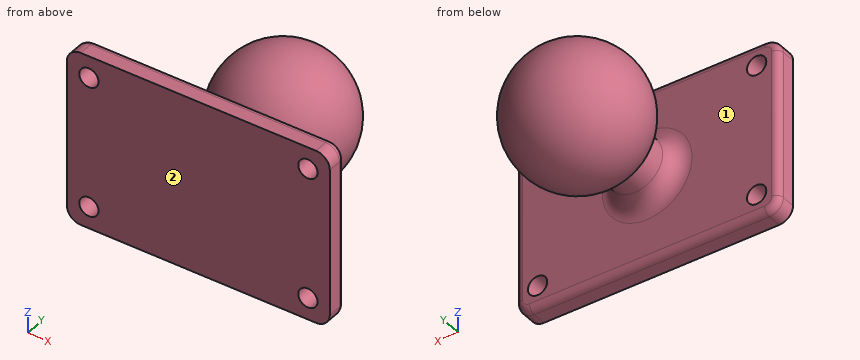
from build123d import *

# Parameters (mm, degrees)
SKETCH1_R           = 2.794
BOSS_EXTRUDE1_DEPTH = 6
FILLET1_R           = 5
FILLET2_R           = 2


with BuildPart() as part:
    # Sketch1 → Boss-Extrude1 (new body)
    with BuildSketch(Plane(origin=(0, 0, 0), x_dir=(1, 0, 0), z_dir=(0, 1, 0))):
        with BuildLine():
            Line((-34.1, -25.4), (34.1, -25.4))
            ThreePointArc((34.1, -25.4), (36.928427125, -24.228427125), (38.1, -21.4))
            Line((38.1, -21.4), (38.1, 21.4))
            ThreePointArc((38.1, 21.4), (36.928427125, 24.228427125), (34.1, 25.4))
            Line((34.1, 25.4), (-34.1, 25.4))
            ThreePointArc((-34.1, 25.4), (-36.928427125, 24.228427125), (-38.1, 21.4))
            Line((-38.1, 21.4), (-38.1, -21.4))
            ThreePointArc((-38.1, -21.4), (-36.928427125, -24.228427125), (-34.1, -25.4))
        make_face()
        with Locations(Location((-31.75, 19.05, 0), (0, 0, 270))):
            Circle(SKETCH1_R, mode=Mode.SUBTRACT)
        with Locations(Location((31.75, 19.05, 0), (0, 0, 270))):
            Circle(SKETCH1_R, mode=Mode.SUBTRACT)
        with Locations(Location((31.75, -19.05, 0), (0, 0, 270))):
            Circle(SKETCH1_R, mode=Mode.SUBTRACT)
        with Locations(Location((-31.75, -19.05, 0), (0, 0, 270))):
            Circle(SKETCH1_R, mode=Mode.SUBTRACT)
    extrude(amount=BOSS_EXTRUDE1_DEPTH)

    # Sketch2 → Revolve1 (revolve)
    with BuildSketch(Plane.XY, mode=Mode.PRIVATE) as revolve1_sk:
        with BuildLine():
            Line((0, 6), (0, 54.022796951))
            ThreePointArc((0, 54.022796951), (-18.604489806, 39.068582473), (-8, 17.684))
            Line((-8, 17.684), (-8, 6))
            Line((-8, 6), (0, 6))
        make_face()
    revolve(revolve1_sk.sketch.rotate(Axis((0, 6, 0), (0, 1, 0)), 180), axis=Axis((0, 6, 0), (0, 1, 0)))

    # Fillet1
    fillet1_edges = [part.edges().sort_by_distance(p)[0] for p in [
        (-8, 6, 0),
    ]]
    fillet(fillet1_edges, radius=FILLET1_R)

    # Fillet2
    fillet2_edges = [part.edges().sort_by_distance(p)[0] for p in [
        (-36.928427125, 6, -24.228427125),
        (-38.1, 6, 0),
        (-36.928427125, 6, 24.228427125),
        (0, 6, 25.4),
        (36.928427125, 6, 24.228427125),
        (38.1, 6, 0),
        (36.928427125, 6, -24.228427125),
        (0, 6, -25.4),
    ]]
    fillet(fillet2_edges, radius=FILLET2_R)


solid = part.part
Geometry check sheet. Reference: the model listing, model coordinates, mm. Face numbers are marked on the shaded views. Give positions to 0.01 mm unless a question says otherwise; leave off trailing zeros. Order: outer loops, then holes, each group sorted by start corner. A loop starts at its lowest first (then second) coordinate and runs counter-clockwise, first axis right, second up.
1) Gauge pin test, flat ends, axial feed: pin 1 (6 mm diameter, centred on x = 13, z = -16, fed in from +Y); pin 2 (4 mm diameter, centred on y = 7.5, z = 19, fed in from +X); pin 3 (10 mm diameter, centred on y = 28.5, z = -5, fed in from -X); pin 4 (4.5 mm diameter, centred on x = 31.75, z = 19.05, fed in from -Y). Record the tip position at first contact, or that the pin passes through.
Results are:
pin 1: stops at y = 42.23
pin 2: stops at x = 37.42
pin 3: stops at x = -18.78
pin 4: passes through
2) Draft check along Y on the marked faces 1 and 2. Enter one of: released by +Y, released by -Y, zero draft, split by the parting line, or undercut.
Results are:
face 1: undercut
face 2: released by -Y
3) Material ranges on probe 1 along X at (y, z) = (1, -19); probe 2 along Z at (x, y) = (31, 3); probe 3 along Z at (x, y) = (30, 5), recorded low to high.
Results are:
probe 1: x = -38.1 to -34.54, -28.96 to 28.96, 34.54 to 38.1
probe 2: z = -25.4 to -21.74, -16.36 to 16.36, 21.74 to 25.4
probe 3: z = -25.13 to -21.23, -16.87 to 16.87, 21.23 to 25.13
4) Cross-section at A-A (x = -31.75). Record the boundary of the cut face in (y, z), then the cut area to 3 significant figures.
Results are:
outline: (0, -25.4) - (4, -25.4) arc R2 ccw to (6, -23.4) - (6, -21.84) - (0, -21.84) - close; (0, -16.26) - (6, -16.26) - (6, 16.26) - (0, 16.26) - close; (0, 21.84) - (6, 21.84) - (6, 23.4) arc R2 ccw to (4, 25.4) - (0, 25.4) - close
area: 236 mm2
5) Cross-section at C-C (z = 0). Record the boundary of the cut face in (x, y).
Results are:
outline: (-38.1, 0) - (38.1, 0) - (38.1, 4) arc R2 ccw to (36.1, 6) - (13, 6) arc R5 cw to (8, 11) - (8, 17.68) arc R19.05 ccw (long way) to (-8, 17.68) - (-8, 11) arc R5 cw to (-13, 6) - (-36.1, 6) arc R2 ccw to (-38.1, 4) - close
6) Cross-section at B-B (x = 0). Record the boundary of the cut face in (y, z).
Results are:
outline: (0, -25.4) - (4, -25.4) arc R2 ccw to (6, -23.4) - (6, -13) arc R5 cw to (11, -8) - (17.68, -8) arc R19.05 ccw (long way) to (17.68, 8) - (11, 8) arc R5 cw to (6, 13) - (6, 23.4) arc R2 ccw to (4, 25.4) - (0, 25.4) - close
7) Cross-section at D-D (x = -15). Record the boundary of the cut face in (y, z).
Results are:
outline: (0, -25.4) - (4, -25.4) arc R2 ccw to (6, -23.4) - (6, 23.4) arc R2 ccw to (4, 25.4) - (0, 25.4) - close; circle Ø23.49 at (34.97, 0)
